Geometry: final body of the model. Coordinates: model frame, mm. Face numbers are marked on the shaded views. A direction names the side the tool comes from. Round coordinates to 2 decimals unless told otherwise and drop trailing zeros. Order: outer loops, then holes, each group sorted by start corner. A loop starts at its lowest first (then second) coordinate and runs counter-clockwise, first axis right, second up. Notation, with made-up numbers: (-2, 11) -> (57, 11) arc R19 ccw to (57, 35) -> close; hole circle Ø8 at (-18, 58.5). An arc over 180 degrees is marked (long way). Put each result on its own line as item: value.
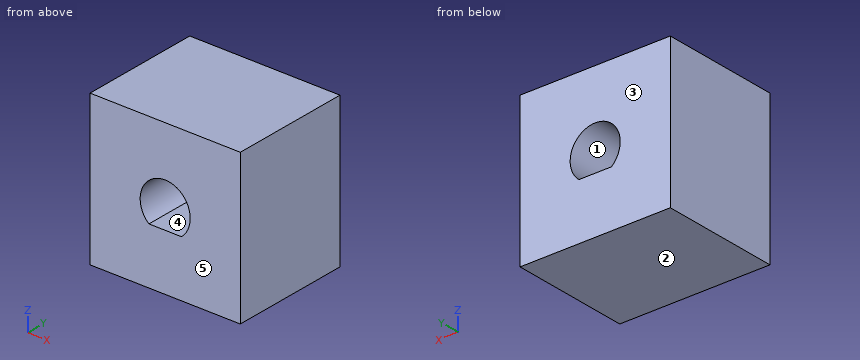
Autodesk Inventor part; units mm, degrees
ref_plane "YZ Plane" through (0, 0, 0) normal (1, 0, 0) x (0, 1, 0)
ref_plane "XZ Plane" through (0, 0, 0) normal (0, 1, 0) x (-1, 0, 0)
ref_plane "XY Plane" through (0, 0, 0) normal (0, 0, 1) x (1, 0, 0)
sketch "Sketch1" plane through (0, 0, 0) normal (0, 1, 0) x (-1, 0, 0)
  line L0 (-9.525, -9.525) -> (9.525, -9.525)
  line L1 (9.525, -9.525) -> (9.525, 9.525)
  line L2 (9.525, 9.525) -> (-9.525, 9.525)
  line L3 (-9.525, 9.525) -> (-9.525, -9.525)
  line L4 (-9.525, -9.525) -> (9.525, 9.525) construction
  line L5 (9.525, -9.525) -> (-9.525, 9.525) construction
  point P0 (0, 0)
  dimension "d0" = 19.05
  dimension "d1" = 19.05
extrude "Extrusion1" add sketch "Sketch1" along normal blind 15.24
sketch "Sketch2" plane through (0, 15.24, 0) normal (0, 1, 0) x (1, 0, 0)
  arc A0 (-2.0635, 2.413) -> (2.0635, 2.413) centre (0, 0) ccw
  line L0 (-2.0635, 2.413) -> (2.0635, 2.413)
  line L1 (-9.525, -9.525) -> (9.525, -9.525)
  dimension "d4" = 6.35
  dimension "d9" = 5.588
extrude "Extrusion2" cut sketch "Sketch2" against normal through all
properties part number "Shaft Connection"
1. Cut plane B-B on z = 0. Return loops of the section in (x, y) (3 decimals).
Ans:
outline: (-9.525, 0) -> (-3.175, 0) -> (-3.175, 15.24) -> (-9.525, 15.24) -> close; (3.175, 0) -> (9.525, 0) -> (9.525, 15.24) -> (3.175, 15.24) -> close
2. Draft query along Z for the marked faces 1, 2 and 3. Return one class per face: +Z half, -Z half, draft (parallel to the pull), parting line (faces both ways), or undercut.
Ans:
face 1: undercut
face 2: -Z half
face 3: draft
3. Set-up query: the marked faces 4 and 5. Return all of +Z, -Z, +X, -X, +Y, -Y with unobstructed straight access to the full face (end or side cutting, diameter ignored); none if empty.
Ans:
face 4: +Y, -Y
face 5: +Z, -Z, +X, -X, -Y
4. Material intervals for probe 1 along Z at (x, y) = (0, 4.25) (3 decimals); probe 2 along Z at (x, y) = (-1.5, 1.25) (3 decimals); probe 3 along X at (y, z) = (5.75, 0.5) (3 decimals), sorted ascending.
Ans:
probe 1: -9.525 to -2.413, 3.175 to 9.525
probe 2: -9.525 to -2.413, 2.798 to 9.525
probe 3: -9.525 to -3.135, 3.135 to 9.525
5. Cut plane A-A on x = 0. Return loops of the section in (y, z) (3 decimals), and give its area (3 significant figures).
Ans:
outline: (0, -9.525) -> (15.24, -9.525) -> (15.24, -2.413) -> (0, -2.413) -> close; (0, 3.175) -> (15.24, 3.175) -> (15.24, 9.525) -> (0, 9.525) -> close
area: 205 mm²
